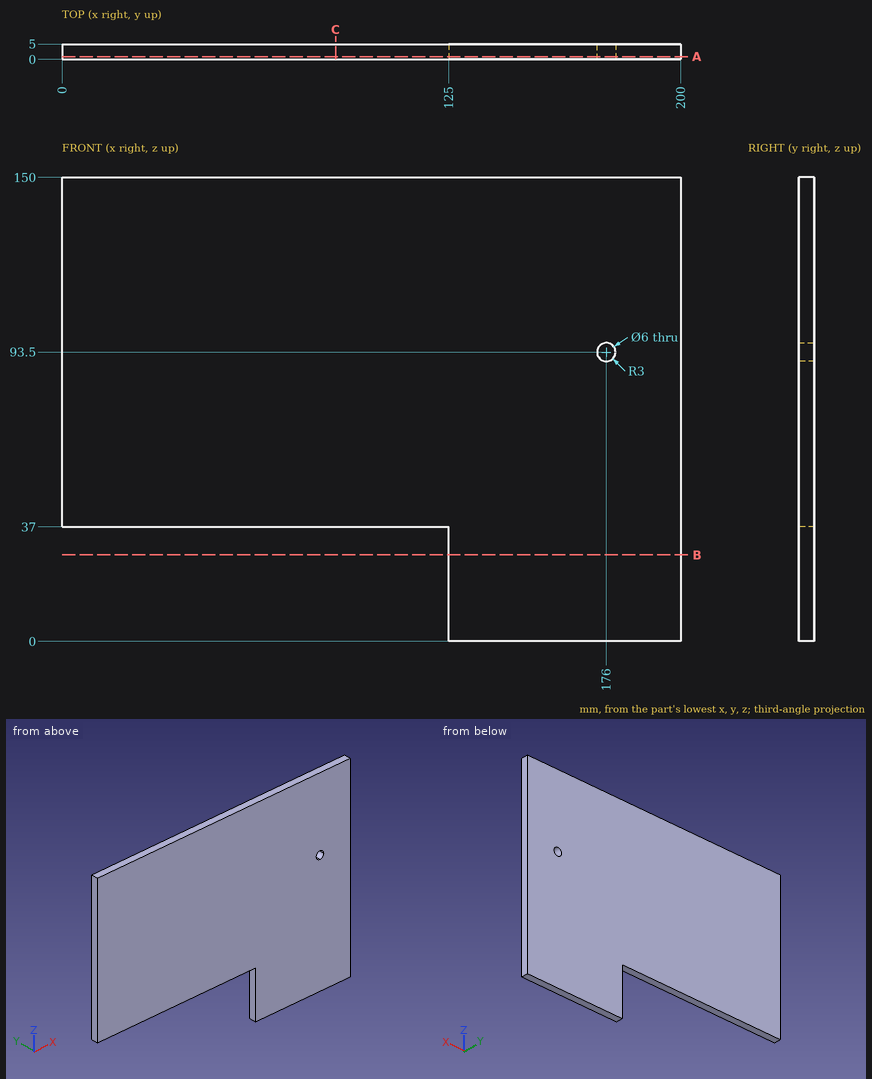
Verification items for this drawing (mm, ordinates from the low corner). Give positions to 0.01 mm unless a question says otherwise; leave off trailing zeros. Order: outer loops, then holes, each group sorted by start corner. A loop starts at its lowest first (then second) coordinate and runs counter-clockwise, first axis right, second up. Notation, with made-up numbers: M -35,-19 L 15,-19 A26 ccw 15,-1 Z; hole C 12.25,-28 d4. An arc over 180 degrees is marked long. Use a Markdown table: item, result.
Item 1: Section check A-A (y = 0.9). Record the cut outline in (x, z), and give its area (3 significant figures).
Answers follow:
| item | result |
|---|---|
| outline | M 0,37 L 125,37 L 125,0 L 200,0 L 200,150 L 0,150 Z; hole C 176,93.5 d6 |
| area | 25,300 mm2 |
Item 2: Depth check by flat-ended pin: P1, Ø2.5, axis at x = 58, y = 1.5, coming from the -Z side. Enter the tip coordinate at first touch or a pass-through.
Answers follow:
| item | result |
|---|---|
| P1 | stops at z = 37 |
Item 3: Section check C-C (x = 88.5). Record the cut outline in (y, z), and give its area (3 significant figures).
Answers follow:
| item | result |
|---|---|
| outline | M 0,37 L 5,37 L 5,150 L 0,150 Z |
| area | 565 mm2 |
Item 4: Material ranges on line 1 along X through (y, z) = (2.85, 93.5); line 2 along Z through (x, y) = (176, 2.4); line 3 along X through (y, z) = (3.95, 33.5), recorded low to high.
Answers follow:
| item | result |
|---|---|
| line 1 | x = 0 to 173, 179 to 200 |
| line 2 | z = 0 to 90.5, 96.5 to 150 |
| line 3 | x = 125 to 200 |
Item 5: Section check B-B (z = 28). Record the cut outline in (x, y), and give its area (3 significant figures).
Answers follow:
| item | result |
|---|---|
| outline | M 125,0 L 200,0 L 200,5 L 125,5 Z |
| area | 375 mm2 |
